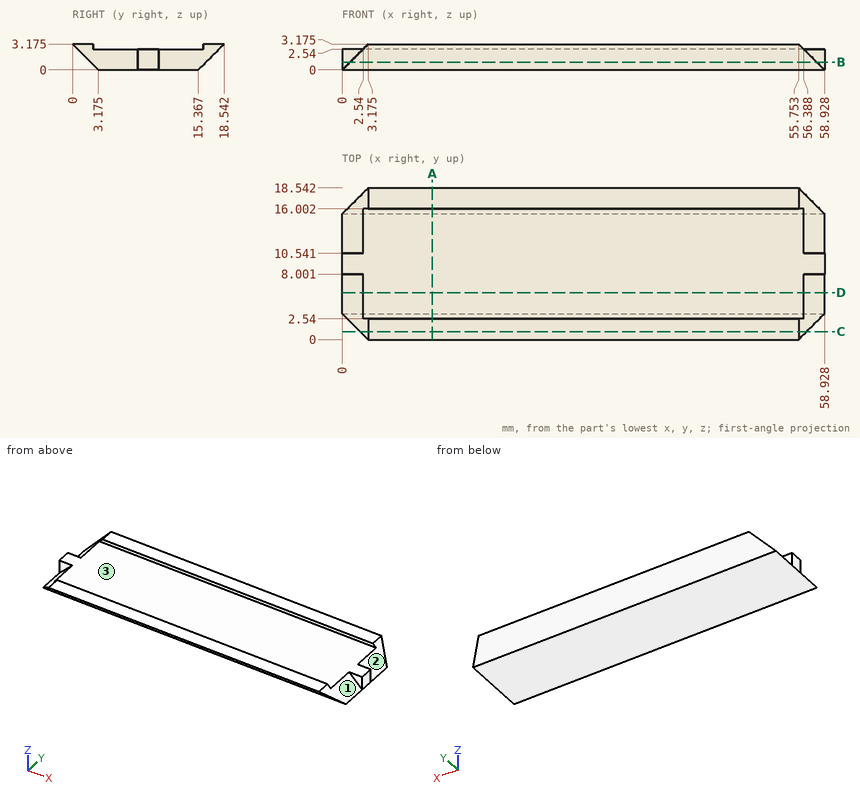
Design review of the part shown in the three views and the two pictorial views. Dimensions are in mm from the part's minimum x, y and z. A direction names the side the tool comes from. Give positions to 0.01 mm unless a question says otherwise; leave off trailing zeros. Loops run counter-clockwise (first coordinate to the right, second up) from the corner with the lowest first, then second, coordinate; pieces in that order, holes last. Notation, with made-up numbers: (18, -1) -> (72, -1) arc R16 cw to (72, 14) -> close; hole circle Ø7 at (74, 4.5). An arc over 180 degrees is marked (long way). Put each result on its own line as item: value. Start each with the question number.
1. We need section B-B on z = 0.95. State the section outline as (x, y) points (3 decimals).
2. Clearance check with flat-ended pins moving along their axes: P1, Ø3, axis at x = 7, y = 7.5, coming from the -Z side; P2, Ø0.8, axis at x = 58, z = 1, coming from the -Y side; P3, Ø1.5, axis at y = 12, z = 1, coming from the +X side; P4, Ø4, axis at x = 35, y = 7.5, coming from the +Z side. State where each tip first meets the part, or that it passes through.
3. We need section A-A on x = 11. State the section outline as (y, z) points (3 decimals), then the cut area to 3 significant figures.
4. We need section C-C on y = 1. State the section outline as (x, z) points (3 decimals), then the cut area to 3 significant figures.
5. We need section D-D on y = 5.75. State the section outline as (x, z) points, then the cut area to 3 significant figures.
6. Wall thickness on probe 1 along Z at (x, y) = (19.5, 14.5); probe 2 along Y at (x, z) = (41, 2.9) (3 decimals); probe 3 along Z at (x, y) = (19.5, 15.75): over which ranges is each line inside the solid? List them lowest first.
7. For the marked faces 1, 2 and 3, list the 3-axis set-ups (+Z, -Z, +X, -X, +Y, -Y) from which the entire face can be reached by the end or side of a thin tool; tool diameter is ignored.
Determined:
1. outline: (0, 8.001) -> (0.95, 8.001) -> (0.95, 2.225) -> (57.978, 2.225) -> (57.978, 8.001) -> (58.928, 8.001) -> (58.928, 10.541) -> (57.978, 10.541) -> (57.978, 16.317) -> (0.95, 16.317) -> (0.95, 10.541) -> (0, 10.541) -> close
2. P1: z = 0
2. P2: y = 1.93
2. P3: x = 58.68
2. P4: z = 2.54
3. outline: (0, 3.175) -> (3.175, 0) -> (15.367, 0) -> (18.542, 3.175) -> (16.002, 3.175) -> (16.002, 2.54) -> (2.54, 2.54) -> (2.54, 3.175) -> close
3. area: 40.2 mm^2
4. outline: (2.175, 2.175) -> (56.753, 2.175) -> (55.753, 3.175) -> (3.175, 3.175) -> close
4. area: 53.6 mm^2
5. outline: (0, 0) -> (58.93, 0) -> (56.39, 2.54) -> (2.54, 2.54) -> close
5. area: 143 mm^2
6. probe 1: 0 to 2.54
6. probe 2: 0.275 to 2.54, 16.002 to 18.267
6. probe 3: 0.38 to 2.54
7. face 1: +Z, +X, -Y
7. face 2: +Z, +X, +Y
7. face 3: +Z, +X, -X
